```python
from build123d import *

# Parameters (mm, degrees)
SKETCH_1_W             = 80
SKETCH_1_H             = 60
SKETCH_1_R             = 2.1
SKETCH_1_R_2           = 1.6
EXTRUDE_2_DEPTH        = 8
SKETCH_1_3_R           = 3
CUT_EXTRUDE_2_DEPTH    = 3.5
FILLET_1_R             = 6
SKETCH_1_4_W           = 35
SKETCH_1_4_H           = 6
CUT_EXTRUDE_3_DEPTH    = 62.395513597
FILLET_2_R             = 3
FILLET_2_OF_MIRROR_1_R = 3
SKETCH_1_5_W           = 8
SKETCH_1_5_H           = 25
CUT_EXTRUDE_4_DEPTH    = 62.395513597
FILLET_3_R             = 4
FILLET_3_OF_MIRROR_2_R = 4
SKETCH_2_R             = 4
CUT_EXTRUDE_5_DEPTH    = 2
SKETCH_3_W             = 30
SKETCH_3_H             = 20
CUT_EXTRUDE_6_DEPTH    = 10
FILLET_4_R             = 10


with BuildPart() as part:
    # 草图1 → 凸台-拉伸2 (new body)
    with BuildSketch(Plane.XY):
        with Locations((-10.979166634, -3.26460069)):
            Rectangle(SKETCH_1_W, SKETCH_1_H)
        with Locations((-40.979166634, 16.73539931)):
            Circle(SKETCH_1_R, mode=Mode.SUBTRACT)
        with Locations(Location((19.020833366, 16.73539931, 0), (0, 0, 180))):
            Circle(SKETCH_1_R, mode=Mode.SUBTRACT)
        with Locations((19.020833366, -23.26460069)):
            Circle(SKETCH_1_R, mode=Mode.SUBTRACT)
        with Locations(Location((-40.979166634, -23.26460069, 0), (0, 0, 180))):
            Circle(SKETCH_1_R, mode=Mode.SUBTRACT)
        with Locations((-18.979166634, 11.73539931)):
            Circle(SKETCH_1_R_2, mode=Mode.SUBTRACT)
        with Locations(Location((-2.979166634, 11.73539931, 0), (0, 0, 180))):
            Circle(SKETCH_1_R_2, mode=Mode.SUBTRACT)
        with Locations((-2.979166634, -18.26460069)):
            Circle(SKETCH_1_R_2, mode=Mode.SUBTRACT)
        with Locations(Location((-18.979166634, -18.26460069, 0), (0, 0, 180))):
            Circle(SKETCH_1_R_2, mode=Mode.SUBTRACT)
    extrude(amount=EXTRUDE_2_DEPTH)

    # 草图1<3> → 切除-拉伸2 (cut)
    with BuildSketch(Plane.XY):
        with Locations((-18.979166634, 11.73539931)):
            Circle(SKETCH_1_3_R)
        with Locations(Location((-2.979166634, 11.73539931, 0), (0, 0, 180))):
            Circle(SKETCH_1_3_R)
        with Locations((-2.979166634, -18.26460069)):
            Circle(SKETCH_1_3_R)
        with Locations(Location((-18.979166634, -18.26460069, 0), (0, 0, 180))):
            Circle(SKETCH_1_3_R)
    extrude(amount=CUT_EXTRUDE_2_DEPTH, mode=Mode.SUBTRACT)

    # 圆角1
    fillet_1_edges = [part.edges().sort_by_distance(p)[0] for p in [
        (-50.979166634, 26.73539931, 4),
        (-50.979166634, -33.26460069, 4),
        (29.020833366, -33.26460069, 4),
        (29.020833366, 26.73539931, 4),
    ]]
    fillet(fillet_1_edges, radius=FILLET_1_R)

    # 草图1<4> → 切除-拉伸3 (cut, through all)
    with BuildSketch(Plane.XY):
        with Locations((-10.979166634, 18.73539931)):
            Rectangle(SKETCH_1_4_W, SKETCH_1_4_H)
    cut_extrude_3 = extrude(amount=CUT_EXTRUDE_3_DEPTH, mode=Mode.SUBTRACT)

    # 圆角2
    fillet_2_edges = [part.edges().sort_by_distance(p)[0] for p in [
        (6.520833366, 15.73539931, 4),
        (6.520833366, 21.73539931, 4),
        (-28.479166634, 15.73539931, 4),
        (-28.479166634, 21.73539931, 4),
    ]]
    fillet(fillet_2_edges, radius=FILLET_2_R - 0.0001)  # a hair under: the kernel refuses the full size

    # 镜向1: 切除-拉伸3 across plane
    add(cut_extrude_3.mirror(Plane.ZX.offset(-3.26460069)), mode=Mode.SUBTRACT)

    # 圆角2 of 镜向1
    fillet_2_of_mirror_1_edges = [part.edges().sort_by_distance(p)[0] for p in [
        (6.520833366, -22.26460069, 4),
        (6.520833366, -28.26460069, 4),
        (-28.479166634, -22.26460069, 4),
        (-28.479166634, -28.26460069, 4),
    ]]
    fillet(fillet_2_of_mirror_1_edges, radius=FILLET_2_OF_MIRROR_1_R - 0.0001)  # a hair under: the kernel refuses the full size

    # 草图1<5> → 切除-拉伸4 (cut, through all)
    with BuildSketch(Plane.XY):
        with Locations((-40.979166634, -3.26460069)):
            Rectangle(SKETCH_1_5_W, SKETCH_1_5_H)
    cut_extrude_4 = extrude(amount=CUT_EXTRUDE_4_DEPTH, mode=Mode.SUBTRACT)

    # 圆角3
    fillet_3_edges = [part.edges().sort_by_distance(p)[0] for p in [
        (-36.979166634, -15.76460069, 4),
        (-44.979166634, -15.76460069, 4),
        (-36.979166634, 9.23539931, 4),
        (-44.979166634, 9.23539931, 4),
    ]]
    fillet(fillet_3_edges, radius=FILLET_3_R - 0.0001)  # a hair under: the kernel refuses the full size

    # 镜向2: 切除-拉伸4 across plane
    add(cut_extrude_4.mirror(Plane.ZY.offset(10.979166634)), mode=Mode.SUBTRACT)

    # 圆角3 of 镜向2
    fillet_3_of_mirror_2_edges = [part.edges().sort_by_distance(p)[0] for p in [
        (15.020833366, -15.76460069, 4),
        (23.020833366, -15.76460069, 4),
        (15.020833366, 9.23539931, 4),
        (23.020833366, 9.23539931, 4),
    ]]
    fillet(fillet_3_of_mirror_2_edges, radius=FILLET_3_OF_MIRROR_2_R - 0.0001)  # a hair under: the kernel refuses the full size

    # 草图2 → 切除-拉伸5 (cut)
    with BuildSketch(Plane.XY.offset(8)):
        with Locations((-40.979166634, 16.73539931)):
            Circle(SKETCH_2_R)
        with Locations(Location((19.020833366, 16.73539931, 0), (0, 0, 180))):
            Circle(SKETCH_2_R)
        with Locations((19.020833366, -23.26460069)):
            Circle(SKETCH_2_R)
        with Locations(Location((-40.979166634, -23.26460069, 0), (0, 0, 180))):
            Circle(SKETCH_2_R)
    extrude(amount=-CUT_EXTRUDE_5_DEPTH, mode=Mode.SUBTRACT)

    # 草图3 → 切除-拉伸6 (cut)
    with BuildSketch(Plane.XY.offset(8)):
        with Locations((-10.979166634, -3.26460069)):
            Rectangle(SKETCH_3_W, SKETCH_3_H)
    extrude(amount=-CUT_EXTRUDE_6_DEPTH, mode=Mode.SUBTRACT)

    # 圆角4
    fillet_4_edges = [part.edges().sort_by_distance(p)[0] for p in [
        (4.020833366, -13.26460069, 4),
        (-25.979166634, -13.26460069, 4),
        (4.020833366, 6.73539931, 4),
        (-25.979166634, 6.73539931, 4),
    ]]
    fillet(fillet_4_edges, radius=FILLET_4_R - 0.0001)  # a hair under: the kernel refuses the full size


solid = part.part
```
Here's how the part is built. I have some questions about the finished solid (model axes, mm). A direction names the side the tool comes from. Coordinates: 2 decimals unless noted, no trailing zeros. Write each loop counter-clockwise with the first axis right and the second up, starting at its lowest first coordinate (ties: lowest second). Pieces come first, ordered by that corner, then holes. Notation, with made-up numbers: (77, -7.5) - (100, -7.5) arc R5 ccw to (100, 0.5) - close; hole circle Ø8 at (-14.5, 84). An arc over 180 degrees is marked (long way). One line per item, written item: value.
1) On a 3-axis mill with a long thin cutter (end or side, diameter ignored), from which of +Z, -Z, +X, -X, +Y, -Y can I reach the whole of each face in a straight line? I mean faces 4 (the flat face through (-20.3, -17, 3.5)), 5 (the flat face through (-43, -22, 6)), 6 (the cylindrical face through (-27.577, 20.88, 4.056)). Say none if no direction works.
Model answer:
face 4: -Z
face 5: +Z
face 6: +Z, -Z
2) I need wall thicknesses on line 1 along X through (y, z) = (-3, 3.25); line 2 along X through (y, z) = (-10.5, 4.5); line 3 along Y through (x, z) = (0, 7). Which ranges of each line are inside material? Lowest first, please.
Model answer:
line 1: x = -50.98 to -44.98, -36.98 to -25.98, 4.02 to 15.02, 23.02 to 29.02
line 2: x = -50.98 to -44.98, -36.98 to -22.88, 0.92 to 15.02, 23.02 to 29.02
line 3: y = -33.26 to -28.26, -22.26 to -11.28, 4.75 to 15.74, 21.74 to 26.74
3) Suppose I cut it at C-C on z = 5. State how many separate pieces and enclosed holes the cut face has, and give its area (3 significant figures).
Model answer:
separate pieces: 1
enclosed holes: 13
area: 3,390 mm²
4) Suppose I cut it at B-B on y = -1. Write out the boundary of the cut face in (x, z), and give its area (3 significant figures).
Model answer:
outline: (-50.98, 0) - (-44.98, 0) - (-44.98, 8) - (-50.98, 8) - close; (-36.98, 0) - (-25.72, 0) - (-25.72, 8) - (-36.98, 8) - close; (3.76, 0) - (15.02, 0) - (15.02, 8) - (3.76, 8) - close; (23.02, 0) - (29.02, 0) - (29.02, 8) - (23.02, 8) - close
area: 276 mm²
5) I'm going to push flat-ended pins straight in: P1, Ø7, axis at x = -40.98, y = -23.26, coming from the +Z side; P2, Ø5.5, axis at x = -18.98, y = -18.26, coming from the -Z side. Where does each tip first touch, or does it pass through?
Model answer:
P1: stops at z = 6
P2: stops at z = 3.5
6) Suppose I cut it at A-A on x = -13. Write out the boundary of the cut face in (y, z), and give its area (3 significant figures).
Model answer:
outline: (-33.26, 0) - (-28.26, 0) - (-28.26, 8) - (-33.26, 8) - close; (-22.26, 0) - (-13.26, 0) - (-13.26, 8) - (-22.26, 8) - close; (6.74, 0) - (15.74, 0) - (15.74, 8) - (6.74, 8) - close; (21.74, 0) - (26.74, 0) - (26.74, 8) - (21.74, 8) - close
area: 224 mm²
7) We'd pull the mould along X, two halves only. Please class faces 1 (the flat face through (-11, -22.265, 4)), 2 (the flat face through (29.021, -4, 4)), 3 (the flat face through (-11, -33.265, 4)): pulls with the +X half, pulls with the -X half, needs draft (parallel to the pull), parting line crosses it, or undercut.
Model answer:
face 1: undercut
face 2: pulls with the +X half
face 3: needs draft
